Check sheet for the modelled part. Datum: model origin and axes. Units: mm. Face numbers are marked on the shaded views. A direction names the side the tool comes from. Coordinates: 2 decimals unless noted, no trailing zeros. Order: outer loops, then holes, each group sorted by start corner. A loop starts at its lowest first (then second) coordinate and runs counter-clockwise, first axis right, second up.
1. Cross-section at A-A (z = 9.75). Enter the section's corners in (x, y), then the cut area to 3 significant figures.
2. Cross-section at B-B (x = -9). Enter the section's corners in (y, z), then the cut area to 3 significant figures.
3. Draft check along Z on the marked faces 6, 7 and 8. Enter one of: released by +Z, released by -Z, zero draft, split by the parting line, or undercut.
4. Gauge pin test, flat ends, axial feed: pin 1 Ø8 at (x, z) = (1, 3.5) entering from -Y; pin 2 Ø6 at (x, y) = (-7, 5.5) entering from +Z; pin 3 Ø1 at (y, z) = (6, -8.5) entering from -X. Record the tip position at first contact, or that the pin passes through.
5. Set-up check for the marked faces 1, 2, 3, 4 and 5: record each of +Z, -Z, +X, -X, +Y, -Y from which the full face is reachable in a straight line by a thin tool's end or side.
6. Thickness scan on line 1 (Z direction, x = 4.75, y = 0.75); line 2 (Z direction, x = -8.5, y = 8.5). Record the ranges inside material, lowest first.
```python
from build123d import *

# Parameters (mm, degrees)
BOSS_EXTRUDE1_DEPTH = 10


with BuildPart() as part:
    # Sketch1 → Boss-Extrude1 (new body)
    with BuildSketch(Plane(origin=(0, 0, 0), x_dir=(1, 0, 0), z_dir=(0, 1, 0))):
        with BuildLine():
            Line((-1.5, 10.75), (1.5, 10.75))
            Line((1.5, 10.75), (2.408073523, 7.890733927))
            ThreePointArc((2.408073523, 7.890733927), (3.157138317, 7.622006143), (3.87682635, 7.282356586))
            Line((3.87682635, 7.282356586), (6.540737726, 8.66205807))
            Line((6.540737726, 8.66205807), (8.66205807, 6.540737726))
            Line((8.66205807, 6.540737726), (7.282356586, 3.87682635))
            ThreePointArc((7.282356586, 3.87682635), (7.622006143, 3.157138317), (7.890733927, 2.408073523))
            Line((7.890733927, 2.408073523), (10.75, 1.5))
            Line((10.75, 1.5), (10.75, -1.5))
            Line((10.75, -1.5), (7.890733927, -2.408073523))
            ThreePointArc((7.890733927, -2.408073523), (7.622006143, -3.157138317), (7.282356586, -3.87682635))
            Line((7.282356586, -3.87682635), (8.66205807, -6.540737726))
            Line((8.66205807, -6.540737726), (6.540737726, -8.66205807))
            Line((6.540737726, -8.66205807), (3.87682635, -7.282356586))
            ThreePointArc((3.87682635, -7.282356586), (3.157138317, -7.622006143), (2.408073523, -7.890733927))
            Line((2.408073523, -7.890733927), (1.5, -10.75))
            Line((1.5, -10.75), (-1.5, -10.75))
            Line((-1.5, -10.75), (-2.408073523, -7.890733927))
            ThreePointArc((-2.408073523, -7.890733927), (-3.157138317, -7.622006143), (-3.87682635, -7.282356586))
            Line((-3.87682635, -7.282356586), (-6.540737726, -8.66205807))
            Line((-6.540737726, -8.66205807), (-8.66205807, -6.540737726))
            Line((-8.66205807, -6.540737726), (-7.282356586, -3.87682635))
            ThreePointArc((-7.282356586, -3.87682635), (-7.622006143, -3.157138317), (-7.890733927, -2.408073523))
            Line((-7.890733927, -2.408073523), (-10.75, -1.5))
            Line((-10.75, -1.5), (-10.75, 1.5))
            Line((-10.75, 1.5), (-7.890733927, 2.408073523))
            ThreePointArc((-7.890733927, 2.408073523), (-7.622006143, 3.157138317), (-7.282356586, 3.87682635))
            Line((-7.282356586, 3.87682635), (-8.66205807, 6.540737726))
            Line((-8.66205807, 6.540737726), (-6.540737726, 8.66205807))
            Line((-6.540737726, 8.66205807), (-3.87682635, 7.282356586))
            ThreePointArc((-3.87682635, 7.282356586), (-3.157138317, 7.622006143), (-2.408073523, 7.890733927))
            Line((-2.408073523, 7.890733927), (-1.5, 10.75))
        make_face()
        with BuildLine():
            Line((0, 4.5), (-0.922144385, 5.422144385))
            ThreePointArc((-0.922144385, 5.422144385), (-1.423504748, 5.312592045), (-1.912471729, 5.156786973))
            Line((-1.912471729, 5.156786973), (-2.25, 3.897114317))
            Line((-2.25, 3.897114317), (-3.509672656, 4.234642588))
            ThreePointArc((-3.509672656, 4.234642588), (-3.889087297, 3.889087297), (-4.234642588, 3.509672656))
            Line((-4.234642588, 3.509672656), (-3.897114317, 2.25))
            Line((-3.897114317, 2.25), (-5.156786973, 1.912471729))
            ThreePointArc((-5.156786973, 1.912471729), (-5.312592045, 1.423504748), (-5.422144385, 0.922144385))
            Line((-5.422144385, 0.922144385), (-4.5, 0))
            Line((-4.5, 0), (-5.422144385, -0.922144385))
            ThreePointArc((-5.422144385, -0.922144385), (-5.312592045, -1.423504748), (-5.156786973, -1.912471729))
            Line((-5.156786973, -1.912471729), (-3.897114317, -2.25))
            Line((-3.897114317, -2.25), (-4.234642588, -3.509672656))
            ThreePointArc((-4.234642588, -3.509672656), (-3.889087297, -3.889087297), (-3.509672656, -4.234642588))
            Line((-3.509672656, -4.234642588), (-2.25, -3.897114317))
            Line((-2.25, -3.897114317), (-1.912471729, -5.156786973))
            ThreePointArc((-1.912471729, -5.156786973), (-1.423504748, -5.312592045), (-0.922144385, -5.422144385))
            Line((-0.922144385, -5.422144385), (0, -4.5))
            Line((0, -4.5), (0.922144385, -5.422144385))
            ThreePointArc((0.922144385, -5.422144385), (1.423504748, -5.312592045), (1.912471729, -5.156786973))
            Line((1.912471729, -5.156786973), (2.25, -3.897114317))
            Line((2.25, -3.897114317), (3.509672656, -4.234642588))
            ThreePointArc((3.509672656, -4.234642588), (3.889087297, -3.889087297), (4.234642588, -3.509672656))
            Line((4.234642588, -3.509672656), (3.897114317, -2.25))
            Line((3.897114317, -2.25), (5.156786973, -1.912471729))
            ThreePointArc((5.156786973, -1.912471729), (5.312592045, -1.423504748), (5.422144385, -0.922144385))
            Line((5.422144385, -0.922144385), (4.5, 0))
            Line((4.5, 0), (5.422144385, 0.922144385))
            ThreePointArc((5.422144385, 0.922144385), (5.312592045, 1.423504748), (5.156786973, 1.912471729))
            Line((5.156786973, 1.912471729), (3.897114317, 2.25))
            Line((3.897114317, 2.25), (4.234642588, 3.509672656))
            ThreePointArc((4.234642588, 3.509672656), (3.889087297, 3.889087297), (3.509672656, 4.234642588))
            Line((3.509672656, 4.234642588), (2.25, 3.897114317))
            Line((2.25, 3.897114317), (1.912471729, 5.156786973))
            ThreePointArc((1.912471729, 5.156786973), (1.423504748, 5.312592045), (0.922144385, 5.422144385))
            Line((0.922144385, 5.422144385), (0, 4.5))
        make_face(mode=Mode.SUBTRACT)
    extrude(amount=BOSS_EXTRUDE1_DEPTH)


solid = part.part
```
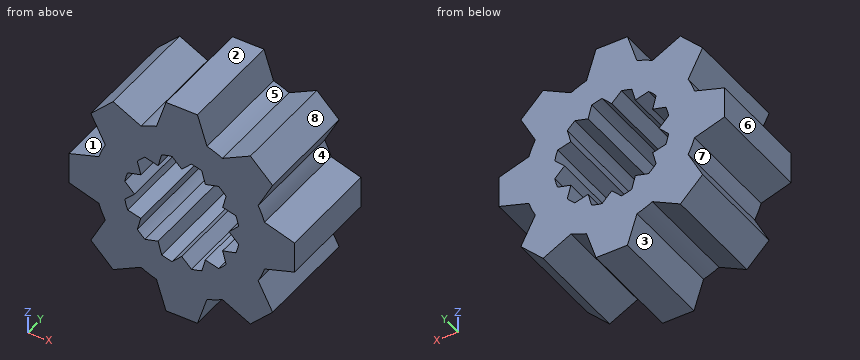
Data:
1. outline: (-1.82, 0) - (1.82, 0) - (1.82, 10) - (-1.82, 10) - close
1. area: 36.4 mm2
2. outline: (0, -2.06) - (10, -2.06) - (10, 2.06) - (0, 2.06) - close
2. area: 41.1 mm2
3. face 6: zero draft
3. face 7: undercut
3. face 8: released by +Z
4. pin 1: stops at y = 0
4. pin 2: stops at z = 8.66
4. pin 3: stops at x = -7.2
5. face 1: -X, +Y, -Y
5. face 2: +Z, +X, -X, +Y, -Y
5. face 3: -Z, +Y, -Y
5. face 4: +X, +Y, -Y
5. face 5: +Z, +Y, -Y
6. line 1: z = -7.73 to -2.02, -0.25 to 0.25, 2.02 to 7.73
6. line 2: z = -6.7 to -6.23, -2.21 to 2.21, 6.23 to 6.7
